from build123d import *

# Parameters (mm, degrees)
F1_DEPTH = 20
F3_DEPTH = 40


with BuildPart() as f1:
    # F0 (on Top) → F1 (new body)
    with BuildSketch(Plane.XY):
        Polygon((-38.37838, 60), (-38.37838, 0), (61.62162, 0), (121.62162, 60), (101.62162, 60), (101.62162, 160), (-18.37838, 160), (-18.37838, 60), align=None)
        Polygon((121.62162, 60), (61.62162, 0), (61.62162, -100), (121.62162, -100), (121.62162, -80), (221.62162, -80), (221.62162, 40), (121.62162, 40), align=None)
    extrude(amount=F1_DEPTH)

    # F2 (on face) → F3 (join)
    with BuildSketch(Plane.XY.offset(20)):
        Polygon((-38.37838, 20), (-38.37838, 0), (61.62162, 0), (61.62162, -100), (81.62162, -100), (81.62162, 0), (81.62162, 20), align=None)
    extrude(amount=F3_DEPTH)


solid = f1.part
Geometry check sheet. Reference: the model listing, model coordinates, mm. A direction names the side the tool comes from. Give positions to 0.01 mm unless a question says otherwise; leave off trailing zeros. Loops run counter-clockwise (first coordinate to the right, second up) from the corner with the lowest first, then second, coordinate; pieces in that order, holes last.
(1) Section check A-A on z = 10.5. Record the cut outline in (x, y).
From the geometry:
outline: (-38.38, 0) - (61.62, 0) - (61.62, -100) - (121.62, -100) - (121.62, -80) - (221.62, -80) - (221.62, 40) - (121.62, 40) - (121.62, 60) - (101.62, 60) - (101.62, 160) - (-18.38, 160) - (-18.38, 60) - (-38.38, 60) - close
(2) Section check B-B on y = -39. Record the cut outline in (x, z), then the cut area to 3 significant figures.
From the geometry:
outline: (61.62, 0) - (221.62, 0) - (221.62, 20) - (81.62, 20) - (81.62, 60) - (61.62, 60) - close
area: 4,000 mm2
(3) Set-up check for faces 1 (the flat face through (-18.378, 111, 10)), 2 (the flat face through (121.622, -90, 10)), 3 (the flat face through (81.622, -41, 40)): record each of +Z, -Z, +X, -X, +Y, -Y from which the full face is reachable in a straight line by a thin tool's end or side.
From the geometry:
face 1: +Z, -Z, -X, +Y
face 2: +Z, -Z, +X, -Y
face 3: +Z, +X, +Y, -Y
(4) Depth check by flat-ended pin: pin 1 Ø1 at (x, y) = (-7.5, 41.5) entering from -Z; pin 2 Ø22 at (x, z) = (172.5, 10.5) entering from -Y; pin 3 Ø6 at (y, z) = (83, 20) entering from -X; pin 4 Ø18 at (y, z) = (-53, 41) entering from -X. Enter the tip coordinate at first touch or a pass-through.
From the geometry:
pin 1: stops at z = 0
pin 2: stops at y = -80
pin 3: stops at x = -18.38
pin 4: stops at x = 61.62
(5) Thickness scan on L1, parallel to Y at x = 10.5, z = 22.5; L2, parallel to Y at x = 117.5, z = 16. Record the ranges inside material, lowest first.
From the geometry:
L1: y = 0 to 20
L2: y = -100 to 60
(6) Section check C-C on x = 94.5. Record the cut outline in (y, z), then the cut area to 3 significant figures.
From the geometry:
outline: (-100, 0) - (160, 0) - (160, 20) - (-100, 20) - close
area: 5,200 mm2
(7) Section check D-D on z = 41.5. Record the cut outline in (x, y), then the cut area to 3 significant figures.
From the geometry:
outline: (-38.38, 0) - (61.62, 0) - (61.62, -100) - (81.62, -100) - (81.62, 20) - (-38.38, 20) - close
area: 4,400 mm2
